CAD build for the part. Positions are in the model's coordinates, mm. Face numbers are marked on the shaded views. A direction names the side the tool comes from. Round coordinates to 2 decimals unless told otherwise and drop trailing zeros. Write each loop counter-clockwise with the first axis right and the second up, starting at its lowest first coordinate (ties: lowest second). Pieces come first, ordered by that corner, then holes. Notation, with made-up numbers: M -8,67 L 49,67 A17 cw 49,97 Z; hole C -6.75,12 d11. An arc over 180 degrees is marked long. Write each question's results on one line, items separated by ' | '. Start each with the question number.
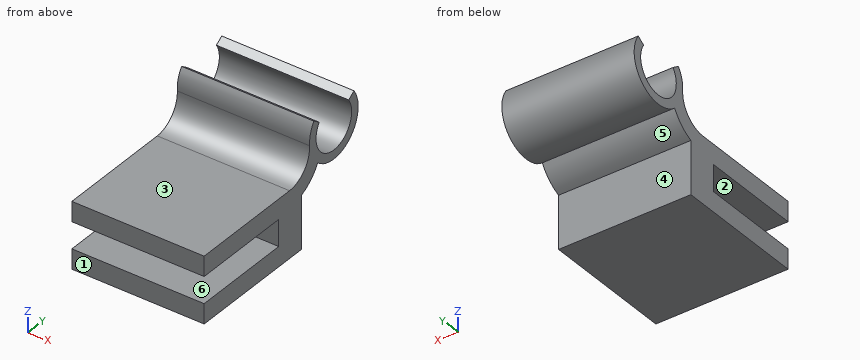
```python
from build123d import *

# Parameters (mm, degrees)
SALIENTE_EXTRUIR1_DEPTH = 15


with BuildPart() as part:
    # Croquis1 → Saliente-Extruir1 (new body, symmetric)
    with BuildSketch(Plane(origin=(0, 0, 0), x_dir=(0, 0, -1), z_dir=(1, 0, 0))):
        with BuildLine():
            Line((-4.485879944, 10.519685039), (7.5, 10.519685039))
            Line((7.5, 10.519685039), (7.5, -19.480314961))
            Line((7.5, -19.480314961), (3, -19.480314961))
            Line((3, -19.480314961), (3, 3.519685039))
            Line((3, 3.519685039), (-3, 3.519685039))
            Line((-3, 3.519685039), (-3, -19.480314961))
            Line((-3, -19.480314961), (-7.5, -19.480314961))
            Line((-7.5, -19.480314961), (-7.5, 6.862248573))
            ThreePointArc((-7.5, 6.862248573), (-9.443341526, 11.362312215), (-14.051551981, 13.033104086))
            ThreePointArc((-14.051551981, 13.033104086), (-16.52030717, 13.29691833), (-18.767660033, 14.35226436))
            Line((-18.767660033, 14.35226436), (-17.629617358, 15.996909874))
            ThreePointArc((-17.629617358, 15.996909874), (-9.000210285, 20.471590491), (-17.550043283, 25.096500086))
            Line((-17.550043283, 25.096500086), (-18.659149931, 26.760796467))
            ThreePointArc((-18.659149931, 26.760796467), (-8.837821951, 25.437991632), (-8.902233659, 15.528191075))
            ThreePointArc((-8.902233659, 15.528191075), (-6.25888029, 13.407663941), (-4.485879944, 10.519685039))
        make_face()
    extrude(amount=SALIENTE_EXTRUIR1_DEPTH, both=True)


solid = part.part
```
1) Saw through at A-A, the plane y = -12.5. Write the cut outline in (x, z), plus the area to 3 significant figures.
2) Saw through at C-C, the plane x = 0.25. Write the cut outline in (y, z), plus the area to 3 significant figures.
3) Wall check: line 1 along Z through (x, y) = (-5.25, -6); line 2 along Y through (x, z) = (2, 14.5); line 3 along Y through (x, z) = (-4.75, -1). Give the ranges that are in metal, low to high. Write a range as from..to.
4) Saw through at B-B, the plane z = -1.25. Write the cut outline in (x, y), plus the area to 3 significant figures.
5) Drop flat-ended pins along their axis: pin 1 Ø5 at (x, z) = (2.5, 1.5) entering from -Y; pin 2 Ø13 at (x, y) = (1.5, -1) entering from +Z; pin 3 Ø6 at (x, z) = (-2.5, 7.5) entering from +Y; pin 4 Ø6 at (x, y) = (10, 18.5) entering from +Z. Give the stop position or say it passes through.
6) Saw through at D-D, the plane y = 8. Write the cut outline in (x, z), plus the area to 3 significant figures.
7) Pull direction Y, two halves, no side cores. Call the marked faces 4, 5 and 6: pulls with the +Y half, pulls with the -Y half, needs draft (parallel to the pull), parting line crosses it, or undercut.
8) 3-axis set-ups, long thin cutter, end or side, ignore diameter. For the marked faces 1, 2 and 3: which of +Z, -Z, +X, -X, +Y, -Y reach the whole face in a straight line?
Filled sheet:
1) outline: M -15,-7.5 L 15,-7.5 L 15,-3 L -15,-3 Z; M -15,3 L 15,3 L 15,7.5 L -15,7.5 Z | area: 270 mm^2
2) outline: M -19.48,-7.5 L 10.52,-7.5 L 10.52,4.49 A9.9 ccw 15.53,8.9 A7.5 ccw 26.76,18.66 L 25.1,17.55 A5.5 cw long 16,17.63 L 14.35,18.77 A7.5 ccw 13.03,14.05 A6.18 cw 6.86,7.5 L -19.48,7.5 L -19.48,3 L 3.52,3 L 3.52,-3 L -19.48,-3 Z | area: 391 mm^2
3) line 1: z = -7.5..-3, 3..7.5 | line 2: y = 13.02..15.02, 26.02..28.02 | line 3: y = 3.52..10.52
4) outline: M -15,3.52 L 15,3.52 L 15,10.52 L -15,10.52 Z | area: 210 mm^2
5) pin 1: stops at y = -19.48 | pin 2: stops at z = 7.5 | pin 3: stops at y = 26.86 | pin 4: stops at z = 17.97
6) outline: M -15,-7.5 L 15,-7.5 L 15,7.61 L -15,7.61 Z | area: 453 mm^2
7) face 4: pulls with the +Y half | face 5: undercut | face 6: needs draft
8) face 1: +Z, -Z, +X, -X, -Y | face 2: +X, -X, -Y | face 3: +Z, +X, -X, -Y
